Autodesk Inventor part; units mm, degrees
ref_plane "YZ Plane" through (0, 0, 0) normal (1, 0, 0) x (0, 1, 0)
ref_plane "XZ Plane" through (0, 0, 0) normal (0, 1, 0) x (-1, 0, 0)
ref_plane "XY Plane" through (0, 0, 0) normal (0, 0, 1) x (1, 0, 0)
sketch "Sketch1" plane through (0, 0, 0) normal (0, 0, 1) x (1, 0, 0)
  line L0 (-31.75, -41.275) -> (31.75, -41.275)
  line L1 (31.75, -41.275) -> (31.75, 41.275)
  line L2 (31.75, 41.275) -> (-31.75, 41.275)
  line L3 (-31.75, 41.275) -> (-31.75, -41.275)
  line L4 (-31.75, -41.275) -> (31.75, 41.275) construction
  line L5 (31.75, -41.275) -> (-31.75, 41.275) construction
  point P0 (0, 0)
  dimension "d0" = 63.5
  dimension "d1" = 82.55
extrude "Extrusion1" add sketch "Sketch1" along normal blind 6.35
sketch "Sketch2" plane through (0, 0, 0) normal (0, 0, -1) x (-1, 0, 0)
  line L0 (44.45, -10) -> (19.05, -10)
  line L1 (19.05, -10) -> (19.05, 10)
  line L2 (19.05, 10) -> (44.45, 10)
  line L3 (44.45, 10) -> (44.45, -10)
  line L4 (31.75, 41.275) -> (31.75, -41.275)
  line L5 (44.45, -10) -> (19.05, 10) construction
  line L6 (19.05, -10) -> (44.45, 10) construction
  point P0 (0, 0)
  point P1 (31.75, 0)
  dimension "d4" = 25.4
  dimension "d5" = 20
extrude "Extrusion2" cut sketch "Sketch2" against normal blind 6.35
sketch "Sketch3" plane through (0, 0, 0) normal (0, 0, -1) x (-1, 0, 0)
  line L0 (25.4, 12.7) -> (25.4, -12.7)
  line L1 (31.75, 41.275) -> (31.75, 10)
  point P0 (0, 0)
  dimension "d8" = 12.7
  dimension "d9" = 25.4
  dimension "d10" = 6.35
hole "Hole1" at (-25.4, 12.7, 0) at (-25.4, -12.7, 0) direction (0, 0, 1) diameter 2.159 end through all
sketch "Sketch4" plane through (0, 0, 0) normal (0, 0, -1) x (-1, 0, 0)
  line L0 (9.525, 28.575) -> (9.525, -28.575)
  line L1 (-31.75, 41.275) -> (31.75, 41.275)
  line L2 (19.05, -10) -> (19.05, 10)
  point P0 (0, 0)
  dimension "d18" = 57.15
  dimension "d19" = 12.7
  dimension "d20" = 9.525
hole "Hole2" at (-9.525, 28.575, 0) at (-9.525, -28.575, 0) direction (0, 0, 1) diameter 4.4958 depth 12.2936 tip angle 118 counterbore diameter 7.9502 counterbore depth 2.54
sketch "Sketch5" plane through (31.75, -41.275, 0) normal (1, 0, 0) x (0, 0, -1)
  line L0 (-3.175, 69.85) -> (-3.175, 12.7)
  line L1 (-6.35, 0) -> (-6.35, 82.55)
  line L2 (0, 82.55) -> (-6.35, 82.55)
  point P0 (0, 41.275)
  dimension "d28" = 57.15
  dimension "d29" = 12.7
  dimension "d30" = 3.175
hole "Hole3" at (31.75, 28.575, 3.175) at (31.75, -28.575, 3.175) direction (-1, 0, 0) diameter 2.6416 depth 10.9728 tip angle 118
properties part number "left side"
Input: part model. Units: mm. Frame: model coordinates. A direction names the side the tool comes from. Give positions to 0.01 mm unless a question says otherwise; leave off trailing zeros. Order: outer loops, then holes, each group sorted by start corner. A loop starts at its lowest first (then second) coordinate and runs counter-clockwise, first axis right, second up.
Q1. Ray query, probe 1 along Y at (x, z) = (-25.4, 1.75) (1 decimal); probe 2 along Y at (x, z) = (-22, 1) (3 decimals); probe 3 along Y at (x, z) = (-8, 2.5) (3 decimals). Return the intervals inside material, ascending.
Checked values:
probe 1: y = -41.3 to -13.8, -11.6 to -10, 10 to 11.6, 13.8 to 41.3
probe 2: y = -41.275 to -10, 10 to 41.275
probe 3: y = -41.275 to -32.246, -24.904 to 24.904, 32.246 to 41.275
Q2. Contact query for flat-ended pins moving along their axis: pin 1 Ø7 at (x, y) = (-9.525, -28.575) entering from +Z; pin 2 Ø2.5 at (y, z) = (-28.575, 3.175) entering from +X; pin 3 Ø4 at (x, y) = (-9.5, -27.5) entering from -Z. Output: stop coordinate, or through.
Checked values:
pin 1: stops at z = 6.35
pin 2: stops at x = 20.73
pin 3: stops at z = 2.54
Q3. Section D-D on y = -5.5. Output: boundary loops of the cut face in (x, z).
Checked values:
outline: (-19.05, 0) - (31.75, 0) - (31.75, 6.35) - (-19.05, 6.35) - close
Q4. Draft query along X for faces 5 (the flat face through (-31.75, 26, 3)), 6 (the cylindrical face through (-26.31, 13.28, 3.22)), 7 (the flat face through (-25, 10, 3)). Return one class per face: +X half, -X half, draft (parallel to the pull), parting line (faces both ways), or undercut.
Checked values:
face 5: -X half
face 6: undercut
face 7: draft
Q5. Section B-B on x = -25.4. State how many separate pieces and enclosed holes the cut face has, and give its area (3 significant figures).
Checked values:
separate pieces: 4
enclosed holes: 0
area: 370 mm2
Q6. Set-up query: faces 1 (the flat face through (0, 1, 0)), 2 (the cylindrical face through (26.187, -29.885, 3.347)), 3 (the cylindrical face through (-9.7, -32.546, 1.288)), 4 (the flat face through (-25, -10, 3)). Return all of +Z, -Z, +X, -X, +Y, -Y with unobstructed straight access to the full face (end or side cutting, diameter ignored); none if empty.
Checked values:
face 1: -Z, +X, -X, +Y, -Y
face 2: +X
face 3: -Z
face 4: +Z, -Z, -X
Q7. Section A-A on y = 12.7. Output: boundary loops of the cut face in (x, z).
Checked values:
outline: (-31.75, 0) - (-26.48, 0) - (-26.48, 6.35) - (-31.75, 6.35) - close; (-24.32, 0) - (31.75, 0) - (31.75, 6.35) - (-24.32, 6.35) - close
